Geometry: final body of the model. Coordinates: model frame, mm. Face numbers are marked on the shaded views. A direction names the side the tool comes from. Coordinates: 2 decimals unless noted, no trailing zeros. Write each loop counter-clockwise with the first axis right and the second up, starting at its lowest first coordinate (ties: lowest second). Pieces come first, ordered by that corner, then holes. Notation, with made-up numbers: (0, 17) -> (53, 17) arc R30 ccw to (53, 43) -> close; hole circle Ø6 at (-6, -29). An arc over 180 degrees is marked (long way). Answer as a JSON object with one key per item and string values. Group by question number.
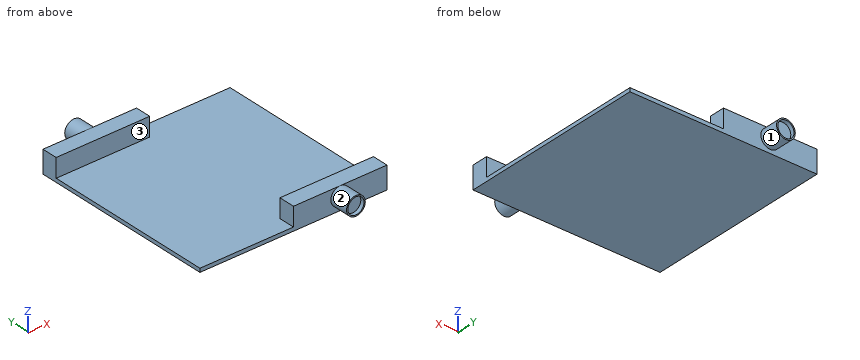
```python
from build123d import *

# Parameters (mm, degrees)
SKETCH1_W           = 150
SKETCH1_H           = 150
BOSS_EXTRUDE1_DEPTH = 3
SKETCH2_R           = 7.5
BOSS_EXTRUDE2_DEPTH = 15
SKETCH4_R           = 7.5
BOSS_EXTRUDE3_DEPTH = 15
SKETCH8_R           = 6.5
CUT_EXTRUDE1_DEPTH  = 3.1
SKETCH9_R           = 6.5
CUT_EXTRUDE2_DEPTH  = 3.1
SKETCH10_W          = 75
SKETCH10_H          = 12.59609842
SKETCH10_H_2        = 12.940455582
BOSS_EXTRUDE4_DEPTH = 15


with BuildPart() as part:
    # Sketch1 → Boss-Extrude1 (new body)
    with BuildSketch(Plane.XY):
        Rectangle(SKETCH1_W, SKETCH1_H)
    extrude(amount=BOSS_EXTRUDE1_DEPTH)



with BuildPart() as body_2:
    # Sketch2 → Boss-Extrude2 (new body)
    with BuildSketch(Plane.XZ.offset(75)):
        with Locations(Location((37.5, 10.5, 0), (0, 0, 270))):
            Circle(SKETCH2_R)
    extrude(amount=BOSS_EXTRUDE2_DEPTH)

    # Sketch8 → Cut-Extrude1 (cut)
    with BuildSketch(Plane.XZ.offset(90)):
        with Locations(Location((37.5, 10.5, 0), (0, 0, 270))):
            Circle(SKETCH8_R)
    extrude(amount=-CUT_EXTRUDE1_DEPTH, mode=Mode.SUBTRACT)


with BuildPart() as body_3:
    # Sketch4 → Boss-Extrude3 (new body)
    with BuildSketch(Plane(origin=(0, 75, 0), x_dir=(1, 0, 0), z_dir=(0, 1, 0))):
        with Locations(Location((-37.5, -10.5, 0), (0, 0, 270))):
            Circle(SKETCH4_R)
    extrude(amount=BOSS_EXTRUDE3_DEPTH)

    # Sketch9 → Cut-Extrude2 (cut)
    with BuildSketch(Plane(origin=(0, 90, 0), x_dir=(1, 0, 0), z_dir=(0, 1, 0))):
        with Locations(Location((-37.5, -10.5, 0), (0, 0, 270))):
            Circle(SKETCH9_R)
    extrude(amount=-CUT_EXTRUDE2_DEPTH, mode=Mode.SUBTRACT)


with BuildPart() as part_1:
    add(part.part)

    add(body_2.part)  # Boss-Extrude4 merges body 2

    add(body_3.part)  # Boss-Extrude4 merges body 3
    # Sketch10 → Boss-Extrude4 (add)
    with BuildSketch(Plane.XY.offset(3)):
        with Locations((-37.5, 68.70195079)):
            Rectangle(SKETCH10_W, SKETCH10_H)
        with Locations((37.5, -68.529772209)):
            Rectangle(SKETCH10_W, SKETCH10_H_2)
    extrude(amount=BOSS_EXTRUDE4_DEPTH)


solid = part_1.part
```
Item 1: Section B-B on y = -70. Output: boundary loops of the cut face in (x, z).
Item 2: Contact query for flat-ended pins moving along their axis: pin 1 (1.5 mm diameter, centred on x = 40.5, y = 56, fed in from -Z); pin 2 (6.5 mm diameter, centred on x = 37.5, z = 11.5, fed in from -Y); pin 3 (6 mm diameter, centred on x = -31, y = -29.5, fed in from +Z); pin 4 (8 mm diameter, centred on x = -37.5, z = 10.5, fed in from +Y). Output: stop coordinate, or through.
Item 3: Section D-D on y = -7. Output: boundary loops of the cut face in (x, z).
Item 4: Section C-C on x = -58.5. Output: boundary loops of the cut face in (y, z), then the cut area to 3 significant figures.
Item 5: Set-up query: the marked faces 1, 2 and 3. Return all of +Z, -Z, +X, -X, +Y, -Y with unobstructed straight access to the full face (end or side cutting, diameter ignored); none if empty.
Item 6: Section A-A on z = 10.5. Output: boundary loops of the cut face in (x, y), then the cut area to 3 significant figures.
Item 7: Ray query, L1, parallel to X at y = 88.55, z = 10.5; L2, parallel to Z at x = -37, y = 87; L3, parallel to X at y = -89.05, z = 10.5. Return the intervals inside material, ascending. Write a range as [from, to].
Answer sheet:
{
 "1": {"outline": "(-75, 0) -> (75, 0) -> (75, 18) -> (0, 18) -> (0, 3) -> (-75, 3) -> close"},
 "2": {"pin 1": "stops at z = 0", "pin 2": "stops at y = -86.9", "pin 3": "stops at z = 3", "pin 4": "stops at y = 86.9"},
 "3": {"outline": "(-75, 0) -> (75, 0) -> (75, 3) -> (-75, 3) -> close"},
 "4": {"outline": "(-75, 0) -> (75, 0) -> (75, 18) -> (62.4, 18) -> (62.4, 3) -> (-75, 3) -> close", "area": "639 mm^2"},
 "5": {"face 1": "+Y", "face 2": "-Y", "face 3": "+Z, +X, -X, -Y"},
 "6": {"outline": "(-75, 62.4) -> (0, 62.4) -> (0, 75) -> (-30, 75) -> (-30, 90) -> (-31, 90) -> (-31, 86.9) -> (-44, 86.9) -> (-44, 90) -> (-45, 90) -> (-45, 75) -> (-75, 75) -> close; (0, -75) -> (30, -75) -> (30, -90) -> (31, -90) -> (31, -86.9) -> (44, -86.9) -> (44, -90) -> (45, -90) -> (45, -75) -> (75, -75) -> (75, -62.06) -> (0, -62.06) -> close", "area": "2,280 mm^2"},
 "7": {"L1": "x = [-45, -44], [-31, -30]", "L2": "z = [3.02, 4.02], [16.98, 17.98]", "L3": "x = [30, 31], [44, 45]"}
}
